Job drawing, mm, ordinate dimensions from the low corner. One solid piece. A direction names the side the tool comes from. Give positions to 0.01 mm unless a question says otherwise; leave off trailing zeros. Order: outer loops, then holes, each group sorted by start corner. A loop starts at its lowest first (then second) coordinate and runs counter-clockwise, first axis right, second up. Notation, with made-up numbers: (27.5, -18.5) - (62.5, -18.5) arc R20 cw to (62.5, -13.5) - close; hole circle Ø6 at (-22, 24.5). An arc over 180 degrees is marked (long way). One line per item, written item: value.
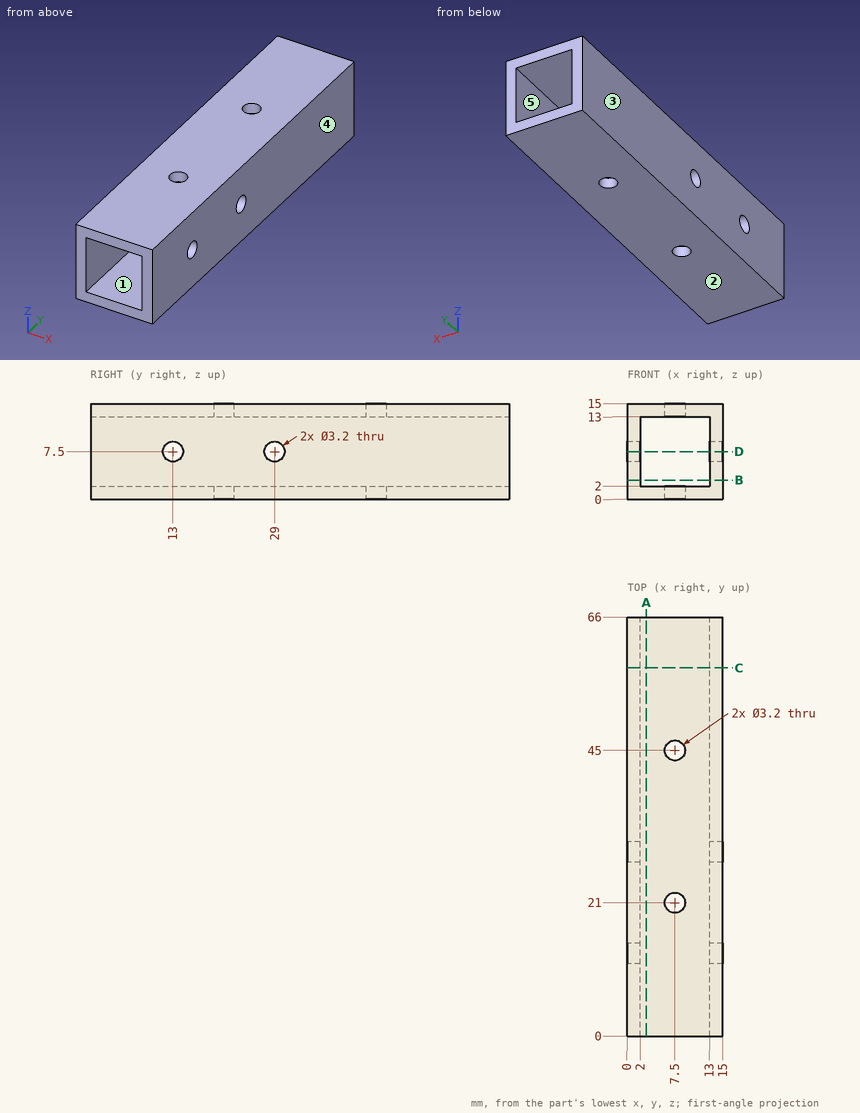
1) Two-plate mould, pull along X, no slides. Class the marked faces 3, 4 and 5: pulls with the +X half, pulls with the -X half, needs draft (parallel to the pull), parting line crosses it, or undercut.
Answer:
face 3: pulls with the -X half
face 4: pulls with the +X half
face 5: undercut
2) Slice it at C-C on y = 58. Write the cut outline in (x, z).
Answer:
outline: (0, 0) - (15, 0) - (15, 15) - (0, 15) - close; hole (2, 2) - (13, 2) - (13, 13) - (2, 13) - close
3) Slice it at A-A on x = 3. Write the cut outline in (y, z).
Answer:
outline: (0, 0) - (66, 0) - (66, 2) - (0, 2) - close; (0, 13) - (66, 13) - (66, 15) - (0, 15) - close
4) Slice it at B-B on z = 3. Write the cut outline in (x, y).
Answer:
outline: (0, 0) - (2, 0) - (2, 66) - (0, 66) - close; (13, 0) - (15, 0) - (15, 66) - (13, 66) - close
5) Slice it at D-D on z = 7.5. Write the cut outline in (x, y).
Answer:
outline: (0, 0) - (2, 0) - (2, 11.4) - (0, 11.4) - close; (0, 14.6) - (2, 14.6) - (2, 27.4) - (0, 27.4) - close; (0, 30.6) - (2, 30.6) - (2, 66) - (0, 66) - close; (13, 0) - (15, 0) - (15, 11.4) - (13, 11.4) - close; (13, 14.6) - (15, 14.6) - (15, 27.4) - (13, 27.4) - close; (13, 30.6) - (15, 30.6) - (15, 66) - (13, 66) - close
6) Drop flat-ended pins along their axis: P1, Ø3.5, axis at y = 13, z = 7.5, coming from the +X side; P2, Ø2.5, axis at x = 7.5, y = 21, coming from the +Z side. Give the stop position or say it passes through.
Answer:
P1: stops at x = 15
P2: passes through
7) Which spindle directions (+Z, -Z, +X, -X, +Y, -Y) get a long thin tool onto all of the face, cutting with end or side? Do the marked faces 1 and 2. Say none if no direction does.
Answer:
face 1: +Y, -Y
face 2: -Z, +X, -X, +Y, -Y
8) Wall check: line 1 along Y through (x, z) = (0.7, 7.5); line 2 along Y through (x, z) = (7.5, 1.4); line 3 along X through (y, z) = (28.5, 5.75). Give the ranges that are in metal, low to high. Write a range as [from, to].
Answer:
line 1: y = [0, 11.4], [14.6, 27.4], [30.6, 66]
line 2: y = [0, 19.4], [22.6, 43.4], [46.6, 66]
line 3: x = [0, 2], [13, 15]
